The model under review builds one solid part; all positions refer to its coordinate system, in mm. Give positions to 0.01 mm unless a question says otherwise; leave off trailing zeros. Loops run counter-clockwise (first coordinate to the right, second up) from the corner with the lowest first, then second, coordinate; pieces in that order, holes last. Notation, with made-up numbers: M 27,-5.5 L 37,-5.5 A17 ccw 37,9.5 Z; hole C -18.5,26 d3. An arc over 180 degrees is marked long. One line per item, written item: value. Start each with the question number.
Q1. We need section C-C on z = 127. Write out the cut boundary in (x, y).
Q2. To check wall thickness, follow line 1 along Y through (x, z) = (0, 104); line 2 along Y through (x, z) = (50, 94.5); line 3 along Z through (x, y) = (-45, -16). State the ranges of each line that lie inside material, in increasing order. Write a range as from..to.
Q3. We need section A-A on y = 0. Write out the cut boundary in (x, z), plus the area to 3 significant figures.
Q4. For pin 1 (10 mm diameter, centred on y = -12, z = 119.5, fed in from +X); pin 2 (3 mm diameter, centred on y = -24, z = 89, fed in from -X); pin 3 (4 mm diameter, centred on y = 13, z = 93.5, fed in from +X), all flat-tipped, find the tip position at first contact; note any pin that passes through.
Q5. Mouldability with a two-part tool opening along X and no side actions: class faces 1 (the face through (-50.4, -38.64, 75.13)), 2 (the face through (-1, 1, 2.54)), 3 (the face through (-13.216, -59.516, 76.421)), 4 (the face through (-1, 1, 0)) as released by +X, released by -X, zero draft, split by the parting line, or undercut.
```python
from build123d import *

# Parameters (mm, degrees)
F0_R     = 63.5059965163
F1_DEPTH = 76.2
F2_T     = -2.54
F3_DEPTH = 76.2


with BuildPart() as f1:
    # F0 (on Top) → F1 (new body)
    with BuildSketch(Plane.XY):
        Circle(F0_R)
    extrude(amount=F1_DEPTH)

    # F2
    f2_openings = [f1.faces().sort_by_distance(p)[0] for p in [
        (0, 0, 76.2),
    ]]
    offset(amount=F2_T, openings=f2_openings)

    # F3 (add): a face of the model
    f3_faces = [f1.faces().sort_by_distance(p)[0] for p in [
        (-61.709775685, 0, 76.2),
    ]]
    extrude(f3_faces, amount=F3_DEPTH)


solid = f1.part
```
Solved:
1. outline: C 0,0 d127.01; hole C 0,0 d121.93
2. line 1: -63.51..-60.97, 60.97..63.51
2. line 2: -39.15..-34.88, 34.88..39.15
2. line 3: 0..2.54
3. outline: M -63.51,0 L 63.51,0 L 63.51,152.4 L 60.97,152.4 L 60.97,2.54 L -60.97,2.54 L -60.97,152.4 L -63.51,152.4 Z
3. area: 1,080 mm2
4. pin 1: x = 63.12
4. pin 2: x = -59.39
4. pin 3: x = 62.55
5. face 1: split by the parting line
5. face 2: undercut
5. face 3: undercut
5. face 4: zero draft
